Source: CAD feature listing. Evaluate the final solid. Frame: model axes, mm. A direction names the side the tool comes from. Coordinates: 2 decimals unless noted, no trailing zeros. Loops run counter-clockwise (first coordinate to the right, second up) from the corner with the lowest first, then second, coordinate; pieces in that order, holes last. Notation, with made-up numbers: (-39, -2.5) -> (-15, -2.5) arc R10 ccw to (-15, 13.5) -> close; hole circle Ø9 at (60, -15.75). An arc over 180 degrees is marked (long way). Answer as a JSON object with one key per item and string values. Group by question number.
from build123d import *

# Parameters (mm, degrees)
F1_DEPTH = 3
F3_DEPTH = 3.4


with BuildPart() as f1:
    # F0 (on Top) → F1 (new body)
    with BuildSketch(Plane.XY):
        with BuildLine():
            ThreePointArc((4.75, 0), (0, -4.75), (-4.75, 0))
            Line((-4.75, 0), (-8.5, 0))
            ThreePointArc((-8.5, 0), (0, -8.5), (8.5, 0))
            Line((8.5, 0), (4.75, 0))
        make_face()
    extrude(amount=F1_DEPTH)

    # F2 (on face) → F3 (join)
    with BuildSketch(Plane.XY.offset(3)):
        with BuildLine():
            Line((-6.2, 0), (-8.5, 0))
            ThreePointArc((-8.5, 0), (0, -8.5), (8.5, 0))
            Line((8.5, 0), (6.2, 0))
            ThreePointArc((6.2, 0), (0, -6.2), (-6.2, 0))
        make_face()
    extrude(amount=F3_DEPTH)


solid = f1.part
1. Section query A-A on y = -3.5. Return loops of the section in (x, z), then the cut area to 3 significant figures.
2. Reachability of faces 1 (the face through (0, -5, 0)), 2 (the face through (0.1, -6.2, 4.7)) from +Z, -Z, +X, -X, +Y, -Y: full face, straight path, thin tool, end or side. Return the list, or none.
3. Mould query, pull axis X, two halves, no side actions, for faces 3 (the face through (-2, -6.1, 6.4)), 4 (the face through (-0.187, -8.498, 3.155)), 5 (the face through (0.1, -4.75, 1.48)). Classes: pulls with the +X half, pulls with the -X half, needs draft (parallel to the pull), parting line crosses it, or undercut.
4. Section query C-C on z = 1. Return loops of the section in (x, y), then the cut area to 3 significant figures.
5. Section query D-D on y = -1.25. Return loops of the section in (x, z), then the cut area to 3 significant figures.
6. Pin query (flat end, axial travel): pin 1 Ø1 at (x, z) = (4, 5.5) entering from +Y (3 decimals); pin 2 Ø2 at (x, z) = (1.5, 3) entering from +Y. Return the tip coordinate at first contact, or that it passes through.
7. Ray query, L1, parallel to Y at x = 0, z = 5.5; L2, parallel to Z at x = 1, y = -6; L3, parallel to X at y = -5, z = 3.25. Return the intervals inside material, ascending.
8. Section query B-B on x = 0. Return loops of the section in (y, z), then the cut area to 3 significant figures.
Solved:
{
 "1": {"outline": "(-7.75, 0) -> (-3.21, 0) -> (-3.21, 3) -> (-5.12, 3) -> (-5.12, 6.4) -> (-7.75, 6.4) -> close; (3.21, 0) -> (7.75, 0) -> (7.75, 6.4) -> (5.12, 6.4) -> (5.12, 3) -> (3.21, 3) -> close", "area": "45.1 mm^2"},
 "2": {"face 1": "-Z, +X, -X, +Y, -Y", "face 2": "+Z, +Y"},
 "3": {"face 3": "needs draft", "face 4": "parting line crosses it", "face 5": "undercut"},
 "4": {"outline": "(-8.5, 0) arc R8.5 ccw to (8.5, 0) -> (4.75, 0) arc R4.75 cw to (-4.75, 0) -> close", "area": "78.0 mm^2"},
 "5": {"outline": "(-8.41, 0) -> (-4.58, 0) -> (-4.58, 3) -> (-6.07, 3) -> (-6.07, 6.4) -> (-8.41, 6.4) -> close; (4.58, 0) -> (8.41, 0) -> (8.41, 6.4) -> (6.07, 6.4) -> (6.07, 3) -> (4.58, 3) -> close", "area": "38.8 mm^2"},
 "6": {"pin 1": "y = -4.265", "pin 2": "y = -4.04"},
 "7": {"L1": "-8.5 to -6.2", "L2": "0 to 3", "L3": "-6.87 to -3.67, 3.67 to 6.87"},
 "8": {"outline": "(-8.5, 0) -> (-4.75, 0) -> (-4.75, 3) -> (-6.2, 3) -> (-6.2, 6.4) -> (-8.5, 6.4) -> close", "area": "19.1 mm^2"}
}
